from build123d import *

# Parameters (mm, degrees)
SKETCH1_W           = 16.3
SKETCH1_H           = 35
SKETCH1_R           = 1.5
BOSS_EXTRUDE1_DEPTH = 8
SKETCH2_W           = 48.4
SKETCH2_H           = 50
BOSS_EXTRUDE2_DEPTH = 8
SKETCH3_R           = 1.75
CUT_EXTRUDE1_DEPTH  = 4
SKETCH4_R           = 1.75
CUT_EXTRUDE2_DEPTH  = 5
SKETCH5_R           = 3
CUT_EXTRUDE3_DEPTH  = 3.2
FILLET1_R           = 4
FILLET2_R           = 3


with BuildPart() as part:
    # Sketch1 → Boss-Extrude1 (new body)
    with BuildSketch(Plane.XY):
        with Locations((322.740686013, 351.682010011)):
            Rectangle(SKETCH1_W, SKETCH1_H)
        with Locations((325.190686013, 343.382010011)):
            Circle(SKETCH1_R, mode=Mode.SUBTRACT)
    extrude(amount=BOSS_EXTRUDE1_DEPTH)

    # Sketch2 → Boss-Extrude2 (add)
    with BuildSketch(Plane(origin=(0, 334.182010011, 0), x_dir=(-1, 0, 0), z_dir=(0, -1, 0))):
        with Locations((-313.481750966, 17)):
            Rectangle(SKETCH2_W, SKETCH2_H)
        with BuildLine():
            Line((-322.681750966, 38), (-304.281750966, 38))
            ThreePointArc((-304.281750966, 38), (-297.210683154, 35.071067812), (-294.281750966, 28))
            Line((-294.281750966, 28), (-294.281750966, 15))
            ThreePointArc((-294.281750966, 15), (-297.210683154, 7.928932188), (-304.281750966, 5))
            Line((-304.281750966, 5), (-322.681750966, 5))
            ThreePointArc((-322.681750966, 5), (-329.752818778, 7.928932188), (-332.681750966, 15))
            Line((-332.681750966, 15), (-332.681750966, 28))
            ThreePointArc((-332.681750966, 28), (-329.752818778, 35.071067812), (-322.681750966, 38))
        make_face(mode=Mode.SUBTRACT)
    extrude(amount=BOSS_EXTRUDE2_DEPTH)

    # Sketch3 → Cut-Extrude1 (cut)
    with BuildSketch(Plane(origin=(0, 0, -42), x_dir=(-1, 0, 0), z_dir=(0, 0, -1))):
        with Locations((-312.481750966, 330.362434358)):
            Circle(SKETCH3_R)
    extrude(amount=-CUT_EXTRUDE1_DEPTH, mode=Mode.SUBTRACT)

    # Sketch4 → Cut-Extrude2 (cut)
    with BuildSketch(Plane.ZY.offset(-289.281750966)):
        with Locations((-21, 330.202094394)):
            Circle(SKETCH4_R)
    extrude(amount=-CUT_EXTRUDE2_DEPTH, mode=Mode.SUBTRACT)

    # Sketch5 → Cut-Extrude3 (cut)
    with BuildSketch(Plane(origin=(0, 0, 0), x_dir=(-1, 0, 0), z_dir=(0, 0, -1))):
        with Locations((-325.190686013, 343.382010011)):
            Circle(SKETCH5_R)
    extrude(amount=-CUT_EXTRUDE3_DEPTH, mode=Mode.SUBTRACT)

    # Fillet1
    fillet1_edges = [part.edges().sort_by_distance(p)[0] for p in [
        (337.681750966, 330.182010011, -42),
        (337.681750966, 330.182010011, 8),
        (289.281750966, 330.182010011, 8),
        (289.281750966, 330.182010011, -42),
    ]]
    fillet(fillet1_edges, radius=FILLET1_R)

    # Fillet2
    # the kernel refuses this fillet: 3 mm, written as the material it takes off along each edge
    with BuildSketch(Plane(origin=(330.890686013, 376.682010011, 0), x_dir=(-1, 0, 0), z_dir=(0, -1, 0))) as fillet2_piece_1:
        with BuildLine():
            CenterArc((FILLET2_R, -FILLET2_R), FILLET2_R, 90, 90)
            Line((0, -FILLET2_R), (0, 0))
            Line((0, 0), (FILLET2_R, 0))
        make_face()
    extrude(amount=42.5, mode=Mode.SUBTRACT)
    with BuildSketch(Plane(origin=(314.590686013, 334.182010011, 0), x_dir=(0, 0, 1), z_dir=(0, 1, 0))) as fillet2_piece_2:
        with BuildLine():
            CenterArc((FILLET2_R, FILLET2_R), FILLET2_R, 180, 90)
            Line((0, FILLET2_R), (0, 0))
            Line((0, 0), (FILLET2_R, 0))
        make_face()
    extrude(amount=42.5, mode=Mode.SUBTRACT)


solid = part.part
Verification items for the finished model (mm, model axes). A direction names the side the tool comes from. Coordinates: 2 decimals unless noted, no trailing zeros. Write each loop counter-clockwise with the first axis right and the second up, starting at its lowest first coordinate (ties: lowest second). Pieces come first, ordered by that corner, then holes. Notation, with made-up numbers: (30, 30.5) - (65, 30.5) arc R31 cw to (65, 54.5) - close; hole circle Ø2 at (38, 19.25). An arc over 180 degrees is marked (long way). Answer as a JSON object with one key per item and string values.
(1) Cross-section at A-A on z = -18. Record the cut outline in (x, y).
Report:
{"outline": "(289.28, 326.18) - (294.28, 326.18) - (294.28, 334.18) - (289.28, 334.18) - close; (332.68, 326.18) - (337.68, 326.18) - (337.68, 334.18) - (332.68, 334.18) - close"}
(2) Gauge pin test, flat ends, axial feed: pin 1 Ø2.5 at (x, y) = (325.19, 343.38) entering from +Z; pin 2 Ø11.5 at (x, y) = (322, 348.5) entering from -Z; pin 3 Ø1.8 at (x, y) = (325, 344.5) entering from -Z; pin 4 Ø5.5 at (y, z) = (353, 5.5) entering from -X. Record the tip position at first contact, or that the pin passes through.
Report:
{"pin 1": "through", "pin 2": "z = 0", "pin 3": "z = 3.2", "pin 4": "x = 314.59"}
(3) Tool access check on faces 5 (the flat face through (313, 330, -5)), 6 (the flat face through (314.591, 351, 5)), 7 (the flat face through (314, 326.182, -1)), 8 (the cylindrical face through (325.841, 340.453, 1.578)), 9 (the flat face through (330.891, 351, 5)). Record the directions out of +Z, -Z, +X, -X, +Y, -Y that give a thin tool (end or side, any length) a straight path to the whole face; none if there is none.
Report:
{"face 5": "+Y, -Y", "face 6": "+Z, -Z, -X, +Y", "face 7": "+Z, -Z, +X, -X, -Y", "face 8": "-Z", "face 9": "+Z, -Z, +X, +Y"}
(4) Thickness scan on line 1 along Y through (x, z) = (293.3, -21); line 2 along Z through (x, y) = (320, 365); line 3 along Y through (x, z) = (307.5, -38.5). Record the ranges inside material, lowest first.
Report:
{"line 1": "326.18 to 328.45, 331.95 to 334.18", "line 2": "0 to 8", "line 3": "326.18 to 334.18"}
(5) Cross-section at D-D on x = 316.5. Record the cut outline in (y, z), plus the area to 3 significant figures.
Report:
{"outline": "(326.18, -42) - (334.18, -42) - (334.18, -38) - (326.18, -38) - close; (326.18, -5) - (334.18, -5) - (334.18, 0.21) - (369.18, 0.21) - (369.18, 8) - (326.18, 8) - close", "area": "409 mm^2"}
(6) Cross-section at B-B on x = 309.5. Record the cut outline in (y, z), plus the area to 3 significant figures.
Report:
{"outline": "(326.18, -42) - (334.18, -42) - (334.18, -38) - (326.18, -38) - close; (326.18, -5) - (334.18, -5) - (334.18, 8) - (326.18, 8) - close", "area": "136 mm^2"}
(7) Cross-section at C-C on y = 335.5. Record the cut outline in (x, z).
Report:
{"outline": "(314.59, 3) arc R3 ccw to (317.59, 0) - (327.89, 0) arc R3 ccw to (330.89, 3) - (330.89, 8) - (314.59, 8) - close"}
(8) Mould release check, pull along Y, two halves, no side actions. Record for faces 1 (the cylindrical face through (336.54, 330.13, -40.8)), 2 (the cylindrical face through (326.621, 343.833, 5.566)), 3 (the cylindrical face through (291.747, 331.937, -21.228)), 4 (the flat face through (314, 334.182, -1)): pulls with the +Y half, pulls with the -Y half, needs draft (parallel to the pull), parting line crosses it, or undercut.
Report:
{"face 1": "needs draft", "face 2": "undercut", "face 3": "undercut", "face 4": "pulls with the +Y half"}
